The listing builds one solid part. Answer for the finished solid, in the listing's coordinates (mm). Face numbers are marked on the shaded views. A direction names the side the tool comes from. Round coordinates to 2 decimals unless told otherwise and drop trailing zeros. Write each loop counter-clockwise with the first axis right and the second up, starting at its lowest first coordinate (ties: lowest second). Pieces come first, ordered by that corner, then holes.
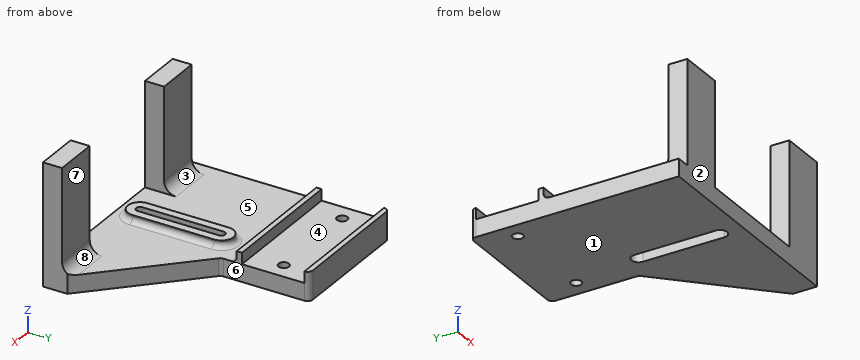
from build123d import *

# Parameters (mm, degrees)
BOSS_EXTRUDE1_DEPTH = 10
SKETCH3_W           = 75
SKETCH3_H           = 3
BOSS_EXTRUDE2_DEPTH = 6.5
SKETCH4_R           = 3
CUT_EXTRUDE2_DEPTH  = 10
SKETCH5_W           = 26
SKETCH5_H           = 11
BOSS_EXTRUDE3_DEPTH = 60
BOSS_EXTRUDE5_DEPTH = 4
CUT_EXTRUDE3_DEPTH  = 186.569394028
FILLET2_START       = -10
FILLET2_DEPTH       = 10
FILLET2_2_DEPTH     = 75
FILLET2_START_2     = -11
FILLET2_3_DEPTH     = 18
CUT_EXTRUDE5_DEPTH  = 7.75
FILLET4_R           = 3
FILLET5_R           = 7


with BuildPart() as part:
    # Sketch2 → Boss-Extrude1 (new body)
    with BuildSketch(Plane.XY):
        Polygon((0, 0), (130, 0), (130, 14), (75, 69), (75, 120), (0, 120), align=None)
    extrude(amount=-BOSS_EXTRUDE1_DEPTH)

    # Sketch3 → Boss-Extrude2 (add)
    with BuildSketch(Plane.XY):
        with Locations((37.5, 118.5)):
            Rectangle(SKETCH3_W, SKETCH3_H)
        with Locations((37.5, 79.5)):
            Rectangle(SKETCH3_W, SKETCH3_H)
    extrude(amount=BOSS_EXTRUDE2_DEPTH)

    # Sketch4 → Cut-Extrude2 (cut)
    with BuildSketch(Plane.XY):
        with Locations((10, 99)):
            Circle(SKETCH4_R)
        with Locations((65, 99)):
            Circle(SKETCH4_R)
    extrude(amount=-CUT_EXTRUDE2_DEPTH, mode=Mode.SUBTRACT)

    # Sketch5 → Boss-Extrude3 (add)
    with BuildSketch(Plane.XY):
        with Locations((117, 5.5)):
            Rectangle(SKETCH5_W, SKETCH5_H)
        with Locations((21, 5.5)):
            Rectangle(SKETCH5_W, SKETCH5_H)
    extrude(amount=BOSS_EXTRUDE3_DEPTH)

    # Sketch7 → Boss-Extrude5 (add)
    with BuildSketch(Plane.XY):
        with BuildLine():
            Line((53, 13), (53, 60))
            ThreePointArc((53, 60), (60, 67), (67, 60))
            Line((67, 60), (67, 13))
            ThreePointArc((67, 13), (60, 6), (53, 13))
        make_face()
    extrude(amount=BOSS_EXTRUDE5_DEPTH)

    # Sketch8 → Cut-Extrude3 (cut, through all)
    with BuildSketch(Plane.XY.offset(4)):
        with BuildLine():
            Line((62.2, 13), (62.2, 60))
            ThreePointArc((62.2, 60), (60, 62.2), (57.8, 60))
            Line((57.8, 60), (57.8, 13))
            ThreePointArc((57.8, 13), (60, 10.8), (62.2, 13))
        make_face()
    extrude(amount=-CUT_EXTRUDE3_DEPTH, mode=Mode.SUBTRACT)

    # Fillet2: read off the stored shape, not the designer's step
    # Fillet2 outline → Fillet2 (add)
    with BuildSketch(Plane.XY.offset(FILLET2_START)):
        with BuildLine():
            ThreePointArc((75.878679656, 68.121320344), (75.228361402, 69.09459039), (75, 70.242640687))
            Line((75, 70.242640687), (75, 69))
            Line((75, 69), (75.878679656, 68.121320344))
        make_face()
    extrude(amount=FILLET2_DEPTH)

    # Fillet2 2 outline → Fillet2 2 (add)
    with BuildSketch(Plane.YZ):
        with BuildLine():
            ThreePointArc((78, 3), (77.121320344, 0.878679656), (75, 0))
            Line((75, 0), (78, 0))
            Line((78, 0), (78, 3))
        make_face()
    extrude(amount=FILLET2_2_DEPTH)

    # Fillet2 3 outline → Fillet2 3 (cut)
    with BuildSketch(Plane.XY.offset(FILLET2_START_2)):
        with BuildLine():
            ThreePointArc((0, 117), (0.878679656, 119.121320344), (3, 120))
            Line((3, 120), (0, 120))
            Line((0, 120), (0, 117))
        make_face()
        with BuildLine():
            ThreePointArc((72, 120), (74.121320344, 119.121320344), (75, 117))
            Line((75, 117), (75, 120))
            Line((75, 120), (72, 120))
        make_face()
    extrude(amount=FILLET2_3_DEPTH, mode=Mode.SUBTRACT)

    # Sketch9 → Cut-Extrude5 (cut)
    with BuildSketch(Plane(origin=(0, 0, -10), x_dir=(-1, 0, 0), z_dir=(0, 0, -1))):
        with BuildLine():
            Line((-64, 60), (-64, 13))
            ThreePointArc((-64, 13), (-60, 9), (-56, 13))
            Line((-56, 13), (-56, 60))
            ThreePointArc((-56, 60), (-60, 64), (-64, 60))
        make_face()
    extrude(amount=-CUT_EXTRUDE5_DEPTH, mode=Mode.SUBTRACT)

    # Fillet4
    fillet4_edges = [part.edges().sort_by_distance(p)[0] for p in [
        (60, 6, 0),
        (67, 36.5, 0),
        (60, 67, 0),
        (53, 36.5, 0),
    ]]
    fillet(fillet4_edges, radius=FILLET4_R)

    # Fillet5
    fillet5_edges = [part.edges().sort_by_distance(p)[0] for p in [
        (117, 11, 0),
        (21, 11, 0),
    ]]
    fillet(fillet5_edges, radius=FILLET5_R)


solid = part.part
1. Section A-A on x = 60 is taken. Determine the outline of the cut face in (y, z), plus the area to 3 significant figures.
Geometry says:
outline: (0, -10) - (9, -10) - (9, -2.25) - (10.8, -2.25) - (10.8, 4) - (6, 4) - (6, 3) arc R3 cw to (3, 0) - (0, 0) - close; (62.2, -2.25) - (64, -2.25) - (64, -10) - (120, -10) - (120, 6.5) - (117, 6.5) - (117, 0) - (81, 0) - (81, 6.5) - (78, 6.5) - (78, 3) arc R3 cw to (75, 0) - (70, 0) arc R3 cw to (67, 3) - (67, 4) - (62.2, 4) - close
area: 741 mm2
2. Given pin 1 (5 mm diameter, centred on y = 84, z = -5, fed in from +X); pin 2 (0.5 mm diameter, centred on y = 45.5, z = 3.5, fed in from -X); pin 3 (2.5 mm diameter, centred on x = 56, y = 79.5, fed in from +Z); pin 4 (3.5 mm diameter, centred on x = 10, y = 99, fed in from -Z), each flat-ended and moving along its own axis, determine where each tip first touches the part or whether it passes through.
Geometry says:
pin 1: stops at x = 75
pin 2: stops at x = 53
pin 3: stops at z = 6.5
pin 4: passes through
3. Straight lines are drawn through the part: line 1 along Z through (x, y) = (69.5, 100); line 2 along Y through (x, z) = (10, -5); line 3 along Y through (x, z) = (105, 25.5). For each, find the intervals that lie inside material, in ascending order.
Geometry says:
line 1: z = -10 to 0
line 2: y = 0 to 96, 102 to 120
line 3: y = 0 to 11
4. A tool of negligible diameter and unlimited length cuts with its end or side. For the marked faces 5, 6, 7 and 8, from which of +Z, -Z, +X, -X, +Y, -Y can it reach the whole face along a straight path? Write none if from no direction.
Geometry says:
face 5: +Z
face 6: +Z, -Z, +X, +Y
face 7: +Z, +X, -X, +Y
face 8: +Z, +X, +Y
5. Section C-C on z = 38.5 is taken. Determine the outline of the cut face in (x, y), plus the area to 3 significant figures.
Geometry says:
outline: (8, 0) - (34, 0) - (34, 11) - (8, 11) - close; (104, 0) - (130, 0) - (130, 11) - (104, 11) - close
area: 572 mm2
6. Section B-B on y = 99 is taken. Determine the outline of the cut face in (x, z), plus the area to 3 significant figures.
Geometry says:
outline: (0, -10) - (7, -10) - (7, 0) - (0, 0) - close; (13, -10) - (62, -10) - (62, 0) - (13, 0) - close; (68, -10) - (75, -10) - (75, 0) - (68, 0) - close
area: 630 mm2
7. Section D-D on y = 55 is taken. Determine the outline of the cut face in (x, z).
Geometry says:
outline: (0, -10) - (56, -10) - (56, -2.25) - (57.8, -2.25) - (57.8, 4) - (53, 4) - (53, 3) arc R3 cw to (50, 0) - (0, 0) - close; (62.2, -2.25) - (64, -2.25) - (64, -10) - (89, -10) - (89, 0) - (70, 0) arc R3 cw to (67, 3) - (67, 4) - (62.2, 4) - close
8. For a pull along Y with two mould halves and no side action, classify the marked faces 1, 2, 3 and 4 as released by +Y, released by -Y, zero draft, split by the parting line, or undercut.
Geometry says:
face 1: zero draft
face 2: released by -Y
face 3: undercut
face 4: undercut
